Autodesk Inventor part; units mm, degrees
ref_plane "L_XY" through (15.2, 0, 0) normal (1, 0, 0) x (0, 0, -1)
ref_plane "L_YZ" through (15.2, 0, 0) normal (0, 0, -1) x (0, 1, 0)
ref_plane "L_ZX" through (15.2, 0, 0) normal (0, 1, 0) x (1, 0, 0)
sketch "Sketch_1" plane through (0, 0, 0) normal (0, 0, 1) x (1, 0, 0)
  line L0 (15.5, 0) -> (0, 0)
  line L1 (0, 0) -> (0, 12.8)
  line L2 (0, 12.8) -> (0.2, 13)
  line L3 (0.2, 13) -> (15.5, 13)
  line L4 (15.5, 13) -> (15.5, 0)
  line L5 (15.5, 0) -> (0, 0)
revolve "Revolution1" add sketch "Sketch_1" angle 360 about axis through (15.5, 0, 0) along (1, 0, 0)
sketch "Sketch_6" plane through (0, 0, 0) normal (1, 0, 0) x (0, 1, 0)
  line L0 (-13, 0.75) -> (-13, -0.75)
  line L1 (-13, -0.75) -> (0, -0.75)
  line L2 (0, -0.75) -> (0, 0.75)
  line L3 (0, 0.75) -> (-13, 0.75)
extrude "Extrusion1" cut sketch "Sketch_6" along normal blind 11.5
sketch "Sketch_7" plane through (5, 0, 0) normal (1, 0, 0) x (0, 0, -1)
  line L0 (-13, -8.4) -> (13, -8.4)
  line L1 (13, -8.4) -> (13, -11.9)
  line L2 (13, -11.9) -> (5, -11.9)
  line L3 (5, -11.9) -> (5, -10.4)
  line L4 (5, -10.4) -> (0.75, -10.4)
  line L5 (0.75, -10.4) -> (0.75, -8.4)
  line L6 (0.75, -8.4) -> (13, -8.4)
revolve "Revolution2" cut sketch "Sketch_7" angle 360 about axis through (5, -8.4, 13) along (0, 0, 1)
sketch "Sketch4" plane through (11.5, 0, 0.75) normal (0, 0, -1) x (-1, 0, 0)
  point P0 (6.5, -8.4)
hole "Hole1" at (5, -8.4, 0.75) direction (0, 0, 1) diameter 3.242 depth 12.25
sketch "Sketch_2" plane through (15.5, 0, 0) normal (1, 0, 0) x (0, 0, -1)
  line L0 (-14, -13.5) -> (14, -13.5)
  line L1 (14, -13.5) -> (14, 13.5)
  line L2 (14, 13.5) -> (-14, 13.5)
  line L3 (-14, 13.5) -> (-14, -13.5)
  line L4 (-13, -3.5) -> (13, -3.5)
  line L5 (13, -3.5) -> (13, 3.5)
  line L6 (13, 3.5) -> (-13, 3.5)
  line L7 (-13, 3.5) -> (-13, -3.5)
extrude "Extrusion2" cut sketch "Sketch_2" against normal blind 4
sketch "Sketch6" plane through (15.5, 0, 0) normal (1, 0, 0) x (0, 0, -1)
  point P0 (0, 0)
hole "Hole2" at (15.5, 0, 0) direction (-1, 0, 0) diameter 13 depth 4
sketch "Sketch_15" plane through (11.5, 0, 0) normal (1, 0, 0) x (0, 0, -1)
  arc A0 (-1, 2.8284) -> (1, 2.8284) centre (0, 0) ccw
  line L0 (1, 2.8284) -> (1, 4)
  line L1 (1, 4) -> (-1, 4)
  line L2 (-1, 4) -> (-1, 2.8284)
extrude "Extrusion3" cut sketch "Sketch_15" along normal mid plane 31
sketch "Sketch_8" plane through (0, 0, 0) normal (1, 0, 0) x (0, 1, 0)
  line L0 (7.155, 0.75) -> (0, 0.75)
  line L1 (0, 0.75) -> (0, -0.75)
  line L2 (0, -0.75) -> (7.155, -0.75)
  line L3 (7.155, -0.75) -> (7.155, 0.75)
extrude "Extrusion4" cut sketch "Sketch_8" along normal blind 15.5
ref_plane "L_XY" through (15.2, 0, 0) normal (1, 0, 0) x (0, 0, -1)
ref_plane "L_YZ" through (15.2, 0, 0) normal (0, 0, -1) x (0, 1, 0)
ref_plane "L_ZX" through (15.2, 0, 0) normal (0, 1, 0) x (1, 0, 0)
ref_plane "screw_XY" through (5, -8.4, -5) normal (0, 0, -1) x (1, 0, 0)
ref_plane "screw_YZ" through (5, -8.4, -5) normal (1, 0, 0) x (0, -1, 0)
ref_plane "screw_ZX" through (5, -8.4, -5) normal (0, -1, 0) x (0, 0, -1)
properties part number "MCOCWK26-6_c"
Verification items for the finished model (mm, model axes). A direction names the side the tool comes from. Round coordinates to 2 decimals unless told otherwise and drop trailing zeros. Write each loop counter-clockwise with the first axis right and the second up, starting at its lowest first coordinate (ties: lowest second). Pieces come first, ordered by that corner, then holes.
1. Draft check along Y on faces 6 (the flat face through (15.5, 0, -9)), 7 (the cylindrical face through (6, 0, -3)), 8 (the flat face through (14, 3.5, 9)), 9 (the flat face through (14, -3.5, 9)). Enter one of: +Y half, -Y half, draft (parallel to the pull), parting line (faces both ways), or undercut.
2. Section check B-B on x = 1. Enter the section's corners in (y, z) (3 decimals), plus the area to 3 significant figures.
3. Access from +Z, -Z, +X, -X, +Y, -Y to the whole of each face (thin tool, end or side, straight path). Record for faces 1 (the flat face through (14, -3.5, -9)), 2 (the cylindrical face through (5.154, -4.903, -7.689)), 3 (the flat face through (5.67, -6.75, 0.75)), 4 (the flat face through (14, 3.5, -9)), 5 (the cylindrical face through (13.5, 0.1, -6.5)).
4. Gauge pin test, flat ends, axial feed: P1, Ø3.5, axis at x = 7, y = 6.5, coming from the +Z side; P2, Ø5, axis at x = 12.5, y = 5, coming from the +Z side; P3, Ø2.5, axis at x = 5, y = -8.4, coming from the -Z side; P4, Ø5, axis at x = 3.5, y = -8, coming from the -Z side. Record the tip position at first contact, or that the pin passes through.
5. Section check C-C on x = 5. Enter the section's corners in (y, z) (3 decimals), plus the area to 3 significant figures.
6. Scan lines: L1, parallel to X at y = -8.4, z = 6.75; L2, parallel to X at y = -8.4, z = -2.95; L3, parallel to Z at x = 7.25, y = 0. Record each from-to range of solid material in increasing order.
7. Section check A-A on y = 0. Enter the section's corners in (x, z).
8. Section check D-D on y = -8.4. State how many separate pieces and enclosed holes the cut face has, plus the area to 3 significant figures.
Answer:
1. face 6: draft
1. face 7: undercut
1. face 8: +Y half
1. face 9: -Y half
2. outline: (-12.978, -0.75) arc R13 ccw (long way) to (-12.978, 0.75) - (-2.905, 0.75) arc R3 cw to (2.828, 1) - (4, 1) - (4, 0.75) - (7.155, 0.75) - (7.155, -0.75) - (4, -0.75) - (4, -1) - (2.828, -1) arc R3 cw to (-2.905, -0.75) - close
2. area: 481 mm2
3. face 1: +Z, -Z, +X, -Y
3. face 2: -Z
3. face 3: +X, -X, -Y
3. face 4: +Z, -Z, +X, +Y
3. face 5: +X
4. P1: stops at z = 12.1
4. P2: stops at z = 12.76
4. P3: passes through
4. P4: stops at z = -11.75
5. outline: (-12.978, -0.75) arc R13 ccw to (-11.9, -5.234) - (-11.9, -5) - (-10.4, -5) - (-10.4, -0.75) - close; (-12.978, 0.75) - (-10.021, 0.75) - (-10.021, 8.281) arc R13 ccw to start; (-6.779, 0.75) - (-2.905, 0.75) arc R3 cw to (2.828, 1) - (4, 1) - (4, 0.75) - (7.155, 0.75) - (7.155, -0.75) - (4, -0.75) - (4, -1) - (2.828, -1) arc R3 cw to (-2.905, -0.75) - (-6.4, -0.75) - (-6.4, -5) - (-4.9, -5) - (-4.9, -12.041) arc R13 ccw (long way) to (-6.779, 11.093) - close
5. area: 403 mm2
6. L1: x = 0 to 3.38, 6.62 to 11.5
6. L2: x = 0 to 3, 7 to 11.5
6. L3: z = -13 to -3, 3 to 13
7. outline: (0, -12.8) - (0.2, -13) - (15.5, -13) - (15.5, -6.5) - (11.5, -6.5) - (11.5, -3) - (0, -3) - close; (0, 3) - (11.5, 3) - (11.5, 6.5) - (15.5, 6.5) - (15.5, 13) - (0.2, 13) - (0, 12.8) - close
8. separate pieces: 4
8. enclosed holes: 0
8. area: 130 mm2
